Study the drawing (mm; zero at the part's minimum x, y, z) and answer. Round coordinates to 2 decimals unless told otherwise and drop trailing zeros. Write each loop counter-clockwise with the first axis right and the second up, starting at its lowest first coordinate (ties: lowest second). Pieces come first, ordered by that corner, then holes. Notation, with made-up numbers: M 60.25,-27 L 118.25,-27 A29 ccw 118.25,3 Z; hole C 65,13.5 d4. An arc over 180 degrees is marked long. Write each question's results on one line, items separated by ' | '.
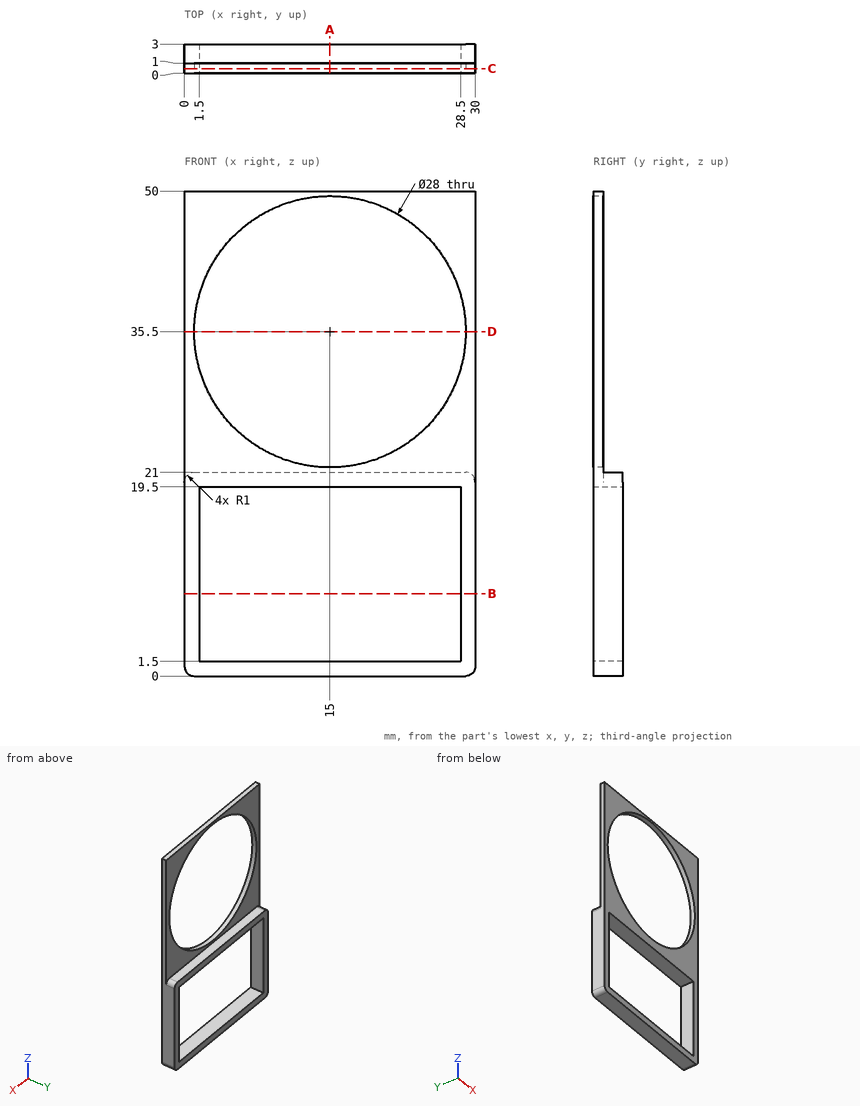
1) This flat-tipped pin is pushed along its axis until it touches: pin 1 (1 mm diameter, centred on x = 17.5, y = 2.5, fed in from +Z). Where does it stop, or does it pass through?
Return value:
pin 1: z = 21
2) Section C-C (y = 0.45) is taken. Determine the outline of the cut face in (x, z).
Return value:
outline: M 0,1 A1 ccw 1,0 L 29,0 A1 ccw 30,1 L 30,50 L 0,50 Z; hole C 15,35.5 d28; hole M 1.5,1.5 L 28.5,1.5 L 28.5,19.5 L 1.5,19.5 Z
3) Section A-A (x = 15) is taken. Determine the outline of the cut face in (y, z), then the cut area to 3 significant figures.
Return value:
outline: M 0,0 L 3,0 L 3,1.5 L 0,1.5 Z; M 0,19.5 L 3,19.5 L 3,21 L 1,21 L 1,21.5 L 0,21.5 Z; M 0,49.5 L 1,49.5 L 1,50 L 0,50 Z | area: 10.0 mm²
4) Section B-B (z = 8.5) is taken. Determine the outline of the cut face in (x, y), then the cut area to 3 significant figures.
Return value:
outline: M 0,0 L 1.5,0 L 1.5,3 L 0,3 Z; M 28.5,0 L 30,0 L 30,3 L 28.5,3 Z | area: 9.00 mm²
5) Section D-D (z = 35.5) is taken. Determine the outline of the cut face in (x, y), then the cut area to 3 significant figures.
Return value:
outline: M 0,0 L 1,0 L 1,1 L 0,1 Z; M 29,0 L 30,0 L 30,1 L 29,1 Z | area: 2.00 mm²
6) Find the intervals of material crossed by line 1 (Z direction, x = 7.25, y = 1.95); line 2 (X direction, y = 0.15, z = 36); line 3 (X direction, y = 0.85, z = 4), in increasing order.
Return value:
line 1: 0 to 1.5, 19.5 to 21 | line 2: 0 to 1.01, 28.99 to 30 | line 3: 0 to 1.5, 28.5 to 30
